```python
from build123d import *

# Parameters (mm, degrees)
ESBO_O2_R                = 15
RESSALTO_EXTRUS_O1_DEPTH = 62
CASCA1_T                 = 3
CORTE_EXTRUS_O2_DEPTH    = 68.02238432


with BuildPart() as part:
    # Esboço2 → Ressalto-extrusão1 (new body)
    with BuildSketch(Plane(origin=(35, 0, 0), x_dir=(0, 0, -1), z_dir=(1, 0, 0))):
        Circle(ESBO_O2_R)
    extrude(amount=-RESSALTO_EXTRUS_O1_DEPTH)

    # Casca1
    casca1_openings = [part.faces().sort_by_distance(p)[0] for p in [
        (35, 0, 0),
        (-27, 0, 0),
    ]]
    offset(amount=CASCA1_T, openings=casca1_openings, kind=Kind.INTERSECTION)

    # Esboço3 → Corte-extrusão2 (cut, through all)
    with BuildSketch(Plane(origin=(35, 0, 0), x_dir=(0, 0, -1), z_dir=(1, 0, 0))):
        with BuildLine():
            Line((-17.2933099, -4.994139836), (17.2933099, -4.994139836))
            ThreePointArc((17.2933099, -4.994139836), (0, -18), (-17.2933099, -4.994139836))
        make_face()
    extrude(amount=-CORTE_EXTRUS_O2_DEPTH, mode=Mode.SUBTRACT)


solid = part.part
```
For this review, take the finished solid that the model builds, in its own axes (mm). Coordinates: 2 decimals unless noted, no trailing zeros. Loops run counter-clockwise (first coordinate to the right, second up) from the corner with the lowest first, then second, coordinate; pieces in that order, holes last.
1. Add section A-A, the plane y = 0. Give the boundary of the cut face in (x, z), then the cut area to 3 significant figures.
2. Mouldability with a two-part tool opening along Z and no side actions: class faces 1 (the cylindrical face through (4, 15, 0)), 2 (the cylindrical face through (4, 18, 0)), 3 (the flat face through (35, 15, -3)) as +Z half, -Z half, draft (parallel to the pull), parting line (faces both ways), or undercut.
3. Add section D-D, the plane z = 5. Give the boundary of the cut face in (x, y), then the cut area to 3 significant figures.
4. For line 1 (Z direction, x = -10, y = 0); line 2 (Y direction, x = -5, z = 0); line 3 (Z direction, x = -2.5, y = 1.75), list the stretches that pass through material, from the lowest coordinate up.
5. Add section B-B, the plane x = -9. Give the boundary of the cut face in (y, z), then the cut area to 3 significant figures.
6. Add section C-C, the plane y = 6.5. Give the boundary of the cut face in (x, z), then the cut area to 3 significant figures.
7. Insertion check: P1, Ø6, axis at x = 22.5, z = -0.5, coming from the -Y side; P2, Ø6, axis at x = -13.5, z = -8.5, coming from the +Y side; P3, Ø6, axis at x = -9.5, y = 8, coming from the -Z side. Each pin has a flat end and moves straight along its axis. Give the tip position at first contact, or say it passes through.
Result:
1. outline: (-27, -18) - (35, -18) - (35, -15) - (-27, -15) - close; (-27, 15) - (35, 15) - (35, 18) - (-27, 18) - close
1. area: 372 mm2
2. face 1: undercut
2. face 2: parting line
2. face 3: draft
3. outline: (-27, 14.14) - (35, 14.14) - (35, 17.29) - (-27, 17.29) - close
3. area: 195 mm2
4. line 1: z = -18 to -15, 15 to 18
4. line 2: y = 15 to 18
4. line 3: z = -17.91 to -14.9, 14.9 to 17.91
5. outline: (-4.99, -17.29) arc R18 ccw (long way) to (-4.99, 17.29) - (-4.99, 14.14) arc R15 cw (long way) to (-4.99, -14.14) - close
5. area: 186 mm2
6. outline: (-27, -16.79) - (35, -16.79) - (35, -13.52) - (-27, -13.52) - close; (-27, 13.52) - (35, 13.52) - (35, 16.79) - (-27, 16.79) - close
6. area: 405 mm2
7. P1: stops at y = 14.59
7. P2: stops at y = 17.14
7. P3: stops at z = -17.29
